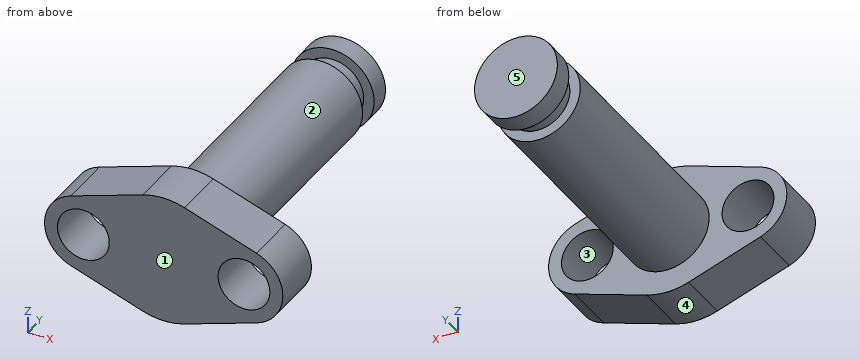
```python
from build123d import *

# Parameters (mm, degrees)
SKETCH1_R           = 2.5
BOSS_EXTRUDE1_DEPTH = 5
SKETCH2_R           = 4
BOSS_EXTRUDE2_DEPTH = 22.5
SKETCH3_R           = 3
BOSS_EXTRUDE3_DEPTH = 2
SKETCH4_R           = 4
BOSS_EXTRUDE4_DEPTH = 2


with BuildPart() as part:
    # Sketch1 → Boss-Extrude1 (new body)
    with BuildSketch(Plane(origin=(0, 0, 0), x_dir=(1, 0, 0), z_dir=(0, 1, 0))):
        with BuildLine():
            ThreePointArc((-2.016129032, -5.9158874), (0, -6.25), (2.016129032, -5.9158874))
            Line((2.016129032, -5.9158874), (8.959677419, -3.54953244))
            ThreePointArc((8.959677419, -3.54953244), (11.5, 0), (8.959677419, 3.54953244))
            Line((8.959677419, 3.54953244), (2.016129032, 5.9158874))
            ThreePointArc((2.016129032, 5.9158874), (0, 6.25), (-2.016129032, 5.9158874))
            Line((-2.016129032, 5.9158874), (-8.959677419, 3.54953244))
            ThreePointArc((-8.959677419, 3.54953244), (-11.5, 0), (-8.959677419, -3.54953244))
            Line((-8.959677419, -3.54953244), (-2.016129032, -5.9158874))
        make_face()
        with Locations(Location((-7.75, 0, 0), (0, 0, 270))):
            Circle(SKETCH1_R, mode=Mode.SUBTRACT)
        with Locations(Location((7.75, 0, 0), (0, 0, 270))):
            Circle(SKETCH1_R, mode=Mode.SUBTRACT)
    extrude(amount=BOSS_EXTRUDE1_DEPTH)

    # Sketch2 → Boss-Extrude2 (add)
    with BuildSketch(Plane(origin=(0, 5, 0), x_dir=(1, 0, 0), z_dir=(0, 1, 0))):
        with Locations(Location((0, 0, 0), (0, 0, 90))):
            Circle(SKETCH2_R)
    extrude(amount=BOSS_EXTRUDE2_DEPTH)

    # Sketch3 → Boss-Extrude3 (add)
    with BuildSketch(Plane(origin=(0, 27.5, 0), x_dir=(1, 0, 0), z_dir=(0, 1, 0))):
        with Locations(Location((0, 0, 0), (0, 0, 270))):
            Circle(SKETCH3_R)
    extrude(amount=BOSS_EXTRUDE3_DEPTH)

    # Sketch4 → Boss-Extrude4 (add)
    with BuildSketch(Plane(origin=(0, 29.5, 0), x_dir=(1, 0, 0), z_dir=(0, 1, 0))):
        with Locations(Location((0, 0, 0), (0, 0, 90))):
            Circle(SKETCH4_R)
    extrude(amount=BOSS_EXTRUDE4_DEPTH)


solid = part.part
```
Input: part model. Units: mm. Frame: model coordinates. Face numbers are marked on the shaded views. A direction names the side the tool comes from. Round coordinates to 2 decimals unless told otherwise and drop trailing zeros. Loops run counter-clockwise (first coordinate to the right, second up) from the corner with the lowest first, then second, coordinate; pieces in that order, holes last. Notation, with made-up numbers: M 82.25,21.5 L 96.25,21.5 A30 cw 96.25,45.5 Z; hole C 10,-36 d3. An arc over 180 degrees is marked long. Answer in a Markdown table with one row per item. Add a question column.
1. Mould query, pull axis X, two halves, no side actions, for the marked faces 3, 4 and 5. Classes: released by +X, released by -X, zero draft, split by the parting line, or undercut.
2. Section A-A (y = 2.5). Output: boundary loops of the cut face in (x, z).
3. Set-up query: the marked faces 1 and 2. Return all of +Z, -Z, +X, -X, +Y, -Y with unobstructed straight access to the full face (end or side cutting, diameter ignored); none if empty.
4. Section B-B (x = 3.5). Output: boundary loops of the cut face in (y, z).
5. Contact query for flat-ended pins moving along their axis: pin 1 (12 mm diameter, centred on x = -0.5, y = 18.5, fed in from -Z); pin 2 (4 mm diameter, centred on x = 3.5, y = 8.5, fed in from +Z); pin 3 (3 mm diameter, centred on y = 18, z = -4.5, fed in from -X). Output: stop coordinate, or through.
6. Section D-D (x = 0). Output: boundary loops of the cut face in (y, z), and give its area (4 significant figures).
7. Ray query, probe 1 along X at (y, z) = (1, 0); probe 2 along Y at (x, z) = (2.25, -3.25); probe 3 along Y at (x, z) = (-2.75, 4.5). Return the intervals inside material, ascending.
8. Section C-C (z = 0). Output: boundary loops of the cut face in (x, y).
Values follow:
| question | item | result |
|---|---|---|
| 1 | face 3 | undercut |
| 1 | face 4 | split by the parting line |
| 1 | face 5 | zero draft |
| 2 | outline | M -8.96,-3.55 L -2.02,-5.92 A6.25 ccw 2.02,-5.92 L 8.96,-3.55 A3.75 ccw 8.96,3.55 L 2.02,5.92 A6.25 ccw -2.02,5.92 L -8.96,3.55 A3.75 ccw Z; hole C -7.75,0 d5; hole C 7.75,0 d5 |
| 3 | face 1 | +Z, -Z, +X, -X, -Y |
| 3 | face 2 | +Y |
| 4 | outline | M 0,-5.41 L 5,-5.41 L 5,-1.94 L 27.5,-1.94 L 27.5,1.94 L 5,1.94 L 5,5.41 L 0,5.41 Z; M 29.5,-1.94 L 31.5,-1.94 L 31.5,1.94 L 29.5,1.94 Z |
| 5 | pin 1 | z = -4 |
| 5 | pin 2 | z = 3.71 |
| 5 | pin 3 | x = -2.65 |
| 6 | outline | M 0,-6.25 L 5,-6.25 L 5,-4 L 27.5,-4 L 27.5,-3 L 29.5,-3 L 29.5,-4 L 31.5,-4 L 31.5,4 L 29.5,4 L 29.5,3 L 27.5,3 L 27.5,4 L 5,4 L 5,6.25 L 0,6.25 Z |
| 6 | area | 270.5 mm^2 |
| 7 | probe 1 | -11.5 to -10.25, -5.25 to 5.25, 10.25 to 11.5 |
| 7 | probe 2 | 0 to 27.5, 29.5 to 31.5 |
| 7 | probe 3 | 0 to 5 |
| 8 | outline | M -11.5,0 L -10.25,0 L -10.25,5 L -11.5,5 Z; M -5.25,0 L 5.25,0 L 5.25,5 L 4,5 L 4,27.5 L 3,27.5 L 3,29.5 L 4,29.5 L 4,31.5 L -4,31.5 L -4,29.5 L -3,29.5 L -3,27.5 L -4,27.5 L -4,5 L -5.25,5 Z; M 10.25,0 L 11.5,0 L 11.5,5 L 10.25,5 Z |
